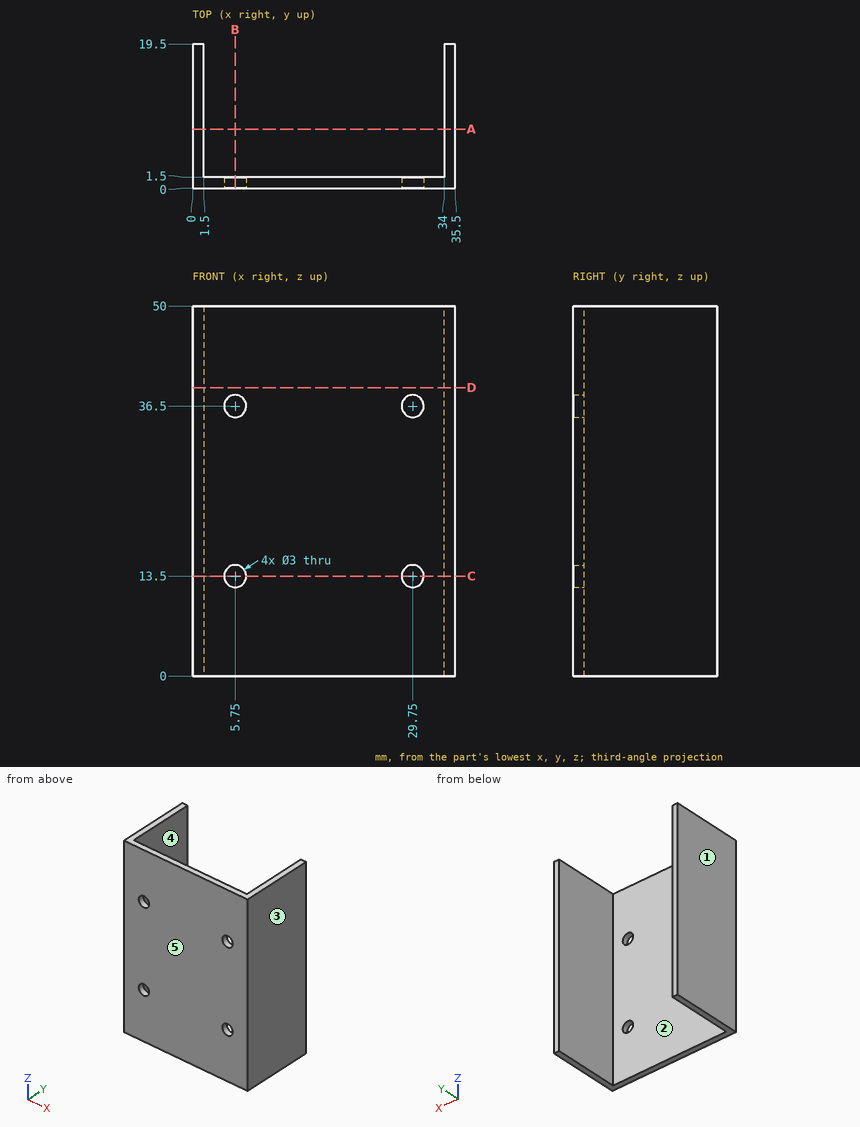
Check sheet for the drawn part. Datum: minimum x, y, z corner. Units: mm. A direction names the side the tool comes from. Give positions to 0.01 mm unless a question says otherwise; leave off trailing zeros. Loops run counter-clockwise (first coordinate to the right, second up) from the corner with the lowest first, then second, coordinate; pieces in that order, holes last.
1) Set-up check for the marked faces 1 and 2: record each of +Z, -Z, +X, -X, +Y, -Y from which the full face is reachable in a straight line by a thin tool's end or side.
2) Depth check by flat-ended pin: pin 1 Ø16 at (x, z) = (18.5, 29) entering from +Y; pin 2 Ø2.5 at (x, z) = (29.75, 36.5) entering from -Y. Enter the tip coordinate at first touch or a pass-through.
3) Sectioned sample at A-A, the plane y = 8. Enter the section's corners in (x, z), then the cut area to 3 significant figures.
4) Draft check along X on the marked faces 3, 4 and 5. Enter one of: pulls with the +X half, pulls with the -X half, needs draft (parallel to the pull), parting line crosses it, or undercut.
5) Sectioned sample at C-C, the plane z = 13.5. Enter the section's corners in (x, y).
6) Thickness scan on line 1 along X through (y, z) = (0.95, 36.5); line 2 along X through (y, z) = (4.5, 39); line 3 along Y through (x, z) = (4, 19). Record the ranges inside material, lowest first.
7) Sectioned sample at B-B, the plane x = 5.75. Enter the section's corners in (y, z), then the cut area to 3 significant figures.
8) Sectioned sample at D-D, the plane z = 39. Enter the section's corners in (x, y).
Answers:
1. face 1: +Z, -Z, -X, +Y, -Y
1. face 2: +Z, -Z, +Y
2. pin 1: stops at y = 1.5
2. pin 2: passes through
3. outline: (0, 0) - (1.5, 0) - (1.5, 50) - (0, 50) - close; (34, 0) - (35.5, 0) - (35.5, 50) - (34, 50) - close
3. area: 150 mm2
4. face 3: pulls with the +X half
4. face 4: undercut
4. face 5: needs draft
5. outline: (0, 0) - (4.25, 0) - (4.25, 1.5) - (1.5, 1.5) - (1.5, 19.5) - (0, 19.5) - close; (7.25, 0) - (28.25, 0) - (28.25, 1.5) - (7.25, 1.5) - close; (31.25, 0) - (35.5, 0) - (35.5, 19.5) - (34, 19.5) - (34, 1.5) - (31.25, 1.5) - close
6. line 1: x = 0 to 4.25, 7.25 to 28.25, 31.25 to 35.5
6. line 2: x = 0 to 1.5, 34 to 35.5
6. line 3: y = 0 to 1.5
7. outline: (0, 0) - (1.5, 0) - (1.5, 12) - (0, 12) - close; (0, 15) - (1.5, 15) - (1.5, 35) - (0, 35) - close; (0, 38) - (1.5, 38) - (1.5, 50) - (0, 50) - close
7. area: 66.0 mm2
8. outline: (0, 0) - (35.5, 0) - (35.5, 19.5) - (34, 19.5) - (34, 1.5) - (1.5, 1.5) - (1.5, 19.5) - (0, 19.5) - close
